Can you work these out from the model? Positions are in its coordinate system, mm. A direction names the side the tool comes from. Give positions to 0.01 mm unless a question says otherwise; leave off trailing zeros. Order: outer loops, then holes, each group sorted by start corner. A loop starts at its lowest first (then second) coordinate and runs counter-clockwise, first axis right, second up. Notation, with made-up numbers: M -14.5,38.25 L 9.5,38.25 A28 cw 9.5,74.25 Z; hole C 7,51.5 d2. An arc over 180 degrees is marked long. Answer as a JSON object with one key per item and string values.
Autodesk Inventor part; units mm, degrees
ref_plane "YZ Plane" through (0, 0, 0) normal (1, 0, 0) x (0, 1, 0)
ref_plane "XZ Plane" through (0, 0, 0) normal (0, 1, 0) x (-1, 0, 0)
ref_plane "XY Plane" through (0, 0, 0) normal (0, 0, 1) x (1, 0, 0)
sketch "Sketch1" plane through (0, 0, 0) normal (0, 0, 1) x (1, 0, 0)
  line L0 (0, 25.4) -> (0, 0)
  line L1 (6.35, -6.35) -> (25.4, -6.35)
  line L2 (31.75, 0) -> (31.75, 25.4)
  line L3 (31.75, 25.4) -> (28.575, 25.4)
  line L4 (28.575, 25.4) -> (28.575, 0)
  line L5 (25.4, -3.175) -> (6.35, -3.175)
  line L6 (3.175, 0) -> (3.175, 25.4)
  line L7 (3.175, 25.4) -> (0, 25.4)
  arc A0 (3.175, 0) -> (6.35, -3.175) centre (6.35, 0) ccw
  arc A1 (0, 0) -> (6.35, -6.35) centre (6.35, 0) ccw
  arc A2 (25.4, -3.175) -> (28.575, 0) centre (25.4, 0) ccw
  arc A3 (25.4, -6.35) -> (31.75, 0) centre (25.4, 0) ccw
  dimension "d0" = 3.175
  dimension "d1" = 25.4
  dimension "d2" = 25.4
  dimension "d3" = 3.175
extrude "Extrusion1" add sketch "Sketch1" along normal blind 101.6
sketch "Sketch2" plane through (31.75, 0, 0) normal (1, 0, 0) x (0, 0, -1)
  line L0 (-101.6, 25.4) -> (-101.6, 0)
  line L1 (0, 25.4) -> (-101.6, 25.4)
  circle A0 centre (-88.9, 12.7) radius 3.175
  dimension "d6" = 6.35
  dimension "d7" = 12.7
  dimension "d8" = 12.7
extrude "Extrusion2" cut sketch "Sketch2" against normal through all
pattern_linear "Rectangular Pattern1" count 7 spacing 25.4 along (0, 0, -1) of "Extrusion2"
sketch "Sketch3" plane through (6.35, -6.35, 0) normal (0, -1, 0) x (1, 0, 0)
  line L0 (19.05, 101.6) -> (0, 101.6)
  circle A0 centre (9.525, 50.8) radius 6.35
  point P0 (-6.35, 0)
  dimension "d14" = 12.7
  dimension "d15" = 50.8
extrude "Extrusion3" cut sketch "Sketch3" against normal up to next
sketch "Sketch4" plane through (6.35, -6.35, 0) normal (0, -1, 0) x (1, 0, 0)
  line L0 (19.05, 101.6) -> (0, 101.6)
  line L1 (0, 0) -> (0, 101.6)
  line L2 (0, 0) -> (19.05, 0)
  line L3 (19.05, 0) -> (19.05, 101.6)
  line L4 (-3.175, 101.6) -> (22.225, 101.6)
  line L5 (22.225, 101.6) -> (22.225, 73.025)
  line L6 (22.225, 73.025) -> (-3.175, 73.025)
  line L7 (-3.175, 73.025) -> (-3.175, 101.6)
  line L8 (-3.175, 165.9576) -> (0, 165.9576) construction
  line L9 (19.05, 165.9576) -> (22.225, 165.9576) construction
  line L10 (-3.175, 0) -> (22.225, 0)
  line L11 (22.225, 0) -> (22.225, 28.575)
  line L12 (22.225, 28.575) -> (-3.175, 28.575)
  line L13 (-3.175, 28.575) -> (-3.175, 0)
  line L14 (-6.35, 101.6) -> (-3.175, 101.6)
  line L15 (-3.175, 101.6) -> (-3.175, 73.025)
  line L16 (-3.175, 73.025) -> (-6.35, 73.025)
  line L17 (-6.35, 73.025) -> (-6.35, 101.6)
  point P0 (-6.35, 0)
  dimension "d18" = 25.4
  dimension "d19" = 28.575
  dimension "d20" = 0
  dimension "d21" = 0
extrude "Extrusion4" cut sketch "Sketch4" against normal through all contours L3 L6 L1 L0 | L4 L5 L6 L3 | L1 L6 L7 L4 | L12 L11 L10 L3 | L3 L2 L1 L12 | L1 L10 L13 L12
properties part number "Frame_OuterConveyorMount" material "Aluminum-6061"
1) Thinking about a two-plate mould opening in Z: for faces 5 (the face through (2, 10, 101.6)), 6 (the face through (2, 25.4, 50)), 7 (the face through (1.61, 12.84, 92.07)), which applies, pulls with the +Z half, pulls with the -Z half, needs draft (parallel to the pull), parting line crosses it, or undercut?
Results found:
{"face 5": "pulls with the +Z half", "face 6": "needs draft", "face 7": "undercut"}
2) I'm going to push flat-ended pins straight in: pin 1 Ø3 at (x, y) = (22, -3) entering from -Z (3 decimals); pin 2 Ø4 at (y, z) = (-3, 50.5) entering from -X; pin 3 Ø1.9 at (x, y) = (13, -3) entering from +Z (3 decimals). Where does each tip first touch, or does it pass through?
Results found:
{"pin 1": "stops at z = 28.575", "pin 2": "stops at x = 0.08", "pin 3": "stops at z = 73.025"}
3) I want a section at C-C on z = 50.8. Write out the boundary of the cut face in (x, y) (3 decimals).
Results found:
{"outline": "M 0,0 A6.35 ccw 6.35,-6.35 L 9.525,-6.35 L 9.525,-3.175 L 6.35,-3.175 A3.175 cw 3.175,0 L 3.175,25.4 L 0,25.4 Z; M 22.225,-6.35 L 25.4,-6.35 A6.35 ccw 31.75,0 L 31.75,25.4 L 28.575,25.4 L 28.575,0 A3.175 cw 25.4,-3.175 L 22.225,-3.175 Z"}
4) For faces 1 (the face through (27.67, -2.22, 50.49)), 2 (the face through (30.641, -3.585, 50.089)), 3 (the face through (16, -5, 28.575)), 4 (the face through (16, -5, 73.025)), which set-ups out of +Z, -Z, +X, -X, +Y, -Y let a thin tool reach every point of the face, with its end or its side?
Results found:
{"face 1": "+Z, -Z, +Y", "face 2": "+Z, -Z, +X, -Y", "face 3": "-Z, +Y, -Y", "face 4": "+Z, +Y, -Y"}
5) I want a section at B-B on y = 5.5. Write out the boundary of the cut face in (x, z) (3 decimals), and give its area (3 significant figures).
Results found:
{"outline": "M 0,0 L 3.175,0 L 3.175,101.6 L 0,101.6 Z; M 28.575,0 L 31.75,0 L 31.75,101.6 L 28.575,101.6 Z", "area": "645 mm²"}
6) I want a section at D-D on x = 16.5. Write out the boundary of the cut face in (y, z) (3 decimals), and give its area (3 significant figures).
Results found:
{"outline": "M -6.35,28.575 L -3.175,28.575 L -3.175,44.481 L -6.35,44.481 Z; M -6.35,57.119 L -3.175,57.119 L -3.175,73.025 L -6.35,73.025 Z", "area": "101 mm²"}
7) I want a section at A-A on z = 88.9. Write out the boundary of the cut face in (x, y) (3 decimals), and give its area (3 significant figures).
Results found:
{"outline": "M 0,0 A6.35 ccw 3.175,-5.499 L 3.175,9.525 L 0,9.525 Z; M 0,15.875 L 3.175,15.875 L 3.175,25.4 L 0,25.4 Z; M 28.575,-5.499 A6.35 ccw 31.75,0 L 31.75,9.525 L 28.575,9.525 Z; M 28.575,15.875 L 31.75,15.875 L 31.75,25.4 L 28.575,25.4 Z", "area": "146 mm²"}
8) I need wall thicknesses on L1, parallel to X at y = 8.5, z = 96 (3 decimals); L2, parallel to Z at x = 30, y = 12; L3, parallel to Y at x = 20, z = 65.5 (3 decimals). Which ranges of each line are inside material? Lowest first, please.
Results found:
{"L1": "x = 0 to 3.175, 28.575 to 31.75", "L2": "z = 0 to 9.6, 15.8 to 35, 41.2 to 60.4, 66.6 to 85.8, 92 to 101.6", "L3": "y = -6.35 to -3.175"}
